Geometry check sheet. Reference: the model listing, model coordinates, mm. Round coordinates to 2 decimals unless told otherwise and drop trailing zeros. Loops run counter-clockwise (first coordinate to the right, second up) from the corner with the lowest first, then second, coordinate; pieces in that order, holes last. Notation, with made-up numbers: (51.5, 61) - (56.5, 61) arc R19 cw to (56.5, 88) - close; hole circle Ø5 at (76.5, 36.5). An arc over 180 degrees is marked (long way). Answer in a Markdown table with one row per item. Add a question column.
```python
from build123d import *

# Parameters (mm, degrees)
BOSS_EXTRUDE1_DEPTH = 1450
FILLET1_START       = -1
FILLET1_DEPTH       = 10
FILLET1_START_2     = 1370
FILLET1_2_DEPTH     = 11


with BuildPart() as part:
    # Sketch1 → Boss-Extrude1 (new body)
    with BuildSketch(Plane.XY):
        with BuildLine():
            Line((1379.522237955, 1177.41513497), (1378.893822938, 1173.464806558))
            ThreePointArc((1378.893822938, 1173.464806558), (428.446906418, 910.229328203), (4.167191444, 19.932197101))
            Line((4.167191444, 19.932197101), (0.167754274, 19.99929645))
            ThreePointArc((0.167754274, 19.99929645), (425.87575598, 913.293505975), (1379.522237955, 1177.41513497))
        make_face()
    extrude(amount=BOSS_EXTRUDE1_DEPTH)

    # Fillet1: read off the stored shape, not the designer's step
    # Fillet1 outline → Fillet1 (cut)
    with BuildSketch(Plane(origin=(0, 0, 0), x_dir=(0.016774837236560897, 0.9998592925185458, 0), z_dir=(0.9998592925185458, -0.016774837236560897, 0)).offset(FILLET1_START)):
        with BuildLine():
            ThreePointArc((119.99929645, 0), (49.288618332, 29.289321882), (19.99929645, 100))
            Line((19.99929645, 100), (19.99929645, 0))
            Line((19.99929645, 0), (119.99929645, 0))
        make_face()
        with BuildLine():
            ThreePointArc((19.99929645, 1350), (49.288618331, 1420.710678119), (119.99929645, 1450))
            Line((119.99929645, 1450), (19.99929645, 1450))
            Line((19.99929645, 1450), (19.99929645, 1350))
        make_face()
    extrude(amount=FILLET1_DEPTH, mode=Mode.SUBTRACT)

    # Fillet1 2 outline → Fillet1 2 (cut)
    with BuildSketch(Plane(origin=(0, 0, 0), x_dir=(0.9875821031103624, -0.15710375430305096, 0), z_dir=(0.15710375430305093, 0.9875821031103625, 0)).offset(FILLET1_START_2)):
        with BuildLine():
            Line((1177.41513497, 0), (1077.41513497, 0))
            ThreePointArc((1077.41513497, 0), (1148.125813089, -29.289321881), (1177.41513497, -100))
            Line((1177.41513497, -100), (1177.41513497, 0))
        make_face()
        with BuildLine():
            Line((1177.41513497, -1450), (1177.41513497, -1350))
            ThreePointArc((1177.41513497, -1350), (1148.125813089, -1420.710678119), (1077.41513497, -1450))
            Line((1077.41513497, -1450), (1177.41513497, -1450))
        make_face()
    extrude(amount=FILLET1_2_DEPTH, mode=Mode.SUBTRACT)


solid = part.part
```
Q1. Cross-section at A-A, the plane z = 121.5. Enter the section's corners in (x, y).
Q2. Scan lines: line 1 (X direction, y = 381.5, z = 679); line 2 (Y direction, x = 396, z = 607); line 3 (Y direction, x = 980.5, z = 167). Record each from-to range of solid material in increasing order. Write a range as from..to.
Q3. Release check for a two-part mould opening along X. For faces 1 (the cylindrical face through (439.408, 919.316, 714.85)), 2 (the cylindrical face through (1349.314, 1178.927, 28.516)) record: +X half, -X half, draft (parallel to the pull), parting line (faces both ways), or undercut.
Q4. Depth check by flat-ended pin: P1, Ø6, axis at y = 452.5, z = 402.5, coming from the +X side; P2, Ø12, axis at y = 647.5, z = 950.5, coming from the +X side; P3, Ø10, axis at y = 825.5, z = 1181.5, coming from the -X side. Enter the tip coordinate at first touch or a pass-through.
Q5. Cross-section at B-B, the plane x = 758.5. Enter the section's corners in (y, z).
Check sheet entries:
| question | item | result |
|---|---|---|
| 1 | outline | (0.17, 20) - (4.17, 19.93) arc R1188.22 cw to (1378.89, 1173.46) - (1379.52, 1177.42) arc R1192.22 ccw to start |
| 2 | line 1 | 62.69..66.91 |
| 2 | line 2 | 881.99..887.37 |
| 2 | line 3 | 1169.21..1173.27 |
| 3 | face 1 | undercut |
| 3 | face 2 | +X half |
| 4 | P1 | x = 94.77 |
| 4 | P2 | x = 199.85 |
| 4 | P3 | x = 327.25 |
| 5 | outline | (1106.23, 0) - (1110.53, 0) - (1110.53, 1450) - (1106.23, 1450) - close |
